Design review of the part shown in the three views and the two pictorial views. Dimensions are in mm from the part's minimum x, y and z. Give positions to 0.01 mm unless a question says otherwise; leave off trailing zeros. Loops run counter-clockwise (first coordinate to the right, second up) from the corner with the lowest first, then second, coordinate; pieces in that order, holes last.
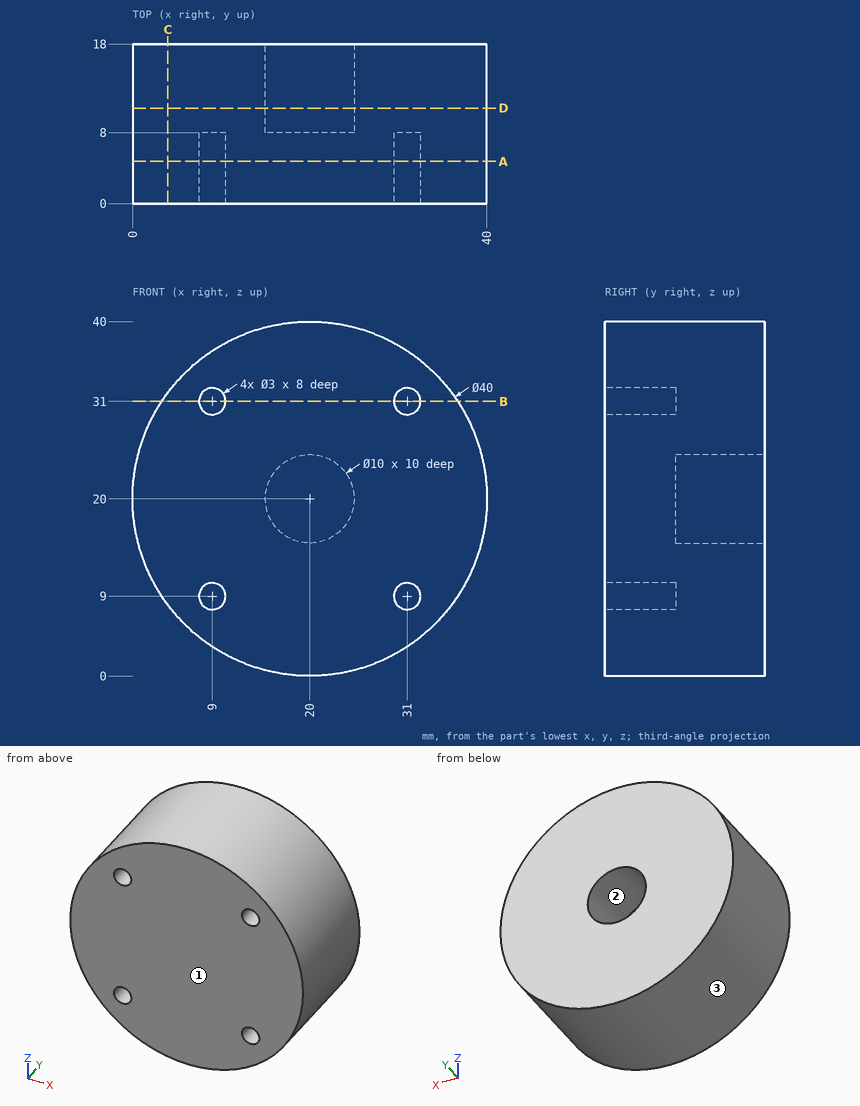
Q1. Take a section at A-A (y = 4.75). Give the boundary of the cut face in (x, z).
Results:
outline: circle Ø40 at (20, 20); hole circle Ø3 at (9, 9); hole circle Ø3 at (9, 31); hole circle Ø3 at (31, 9); hole circle Ø3 at (31, 31)
Q2. Take a section at D-D (y = 10.75). Give the boundary of the cut face in (x, z), plus the area to 3 significant figures.
Results:
outline: circle Ø40 at (20, 20); hole circle Ø10 at (20, 20)
area: 1,180 mm2
Q3. Wall thickness on line 1 (Z direction, x = 30.5, y = 5); line 2 (Z direction, x = 31, y = 5.75); line 3 (X direction, y = 13, z = 20): over which ranges is each line inside the solid? List them lowest first.
Results:
line 1: z = 2.98 to 7.59, 10.41 to 29.59, 32.41 to 37.02
line 2: z = 3.3 to 7.5, 10.5 to 29.5, 32.5 to 36.7
line 3: x = 0 to 15, 25 to 40
Q4. Take a section at B-B (z = 31). Give the boundary of the cut face in (x, y), plus the area to 3 significant figures.
Results:
outline: (3.3, 0) - (7.5, 0) - (7.5, 8) - (10.5, 8) - (10.5, 0) - (29.5, 0) - (29.5, 8) - (32.5, 8) - (32.5, 0) - (36.7, 0) - (36.7, 18) - (3.3, 18) - close
area: 553 mm2
Q5. Take a section at C-C (x = 4). Give the boundary of the cut face in (y, z).
Results:
outline: (0, 8) - (18, 8) - (18, 32) - (0, 32) - close
Q6. Insertion check: pin 1 (1.5 mm diameter, centred on x = 31.5, z = 31, fed in from -Y); pin 2 (4 mm diameter, centred on x = 35, y = 4.5, fed in from -Z); pin 3 (5 mm diameter, centred on x = 19, z = 20.5, fed in from +Y). Each pin has a flat end and moves straight along its axis. Give the tip position at first contact, or say it passes through.
Results:
pin 1: stops at y = 8
pin 2: stops at z = 4.8
pin 3: stops at y = 8
Q7. Draft analysis for pull direction X (two halves, no side actions). For the marked faces 1, 2 and 3, state which applies: pulls with the +X half, pulls with the -X half, needs draft (parallel to the pull), parting line crosses it, or undercut.
Results:
face 1: needs draft
face 2: undercut
face 3: parting line crosses it
